from build123d import *

# Parameters (mm, degrees)
F0_W           = 101.6
F0_H           = 63.5
F1_DEPTH       = 6.35
F2_D           = 3.6576
F2_CSINK_D     = 7.7978
F2_CSINK_ANGLE = 82
F3_R           = 5.08


with BuildPart() as f1:
    # F0 (on Top) → F1 (new body)
    with BuildSketch(Plane.XY):
        Rectangle(F0_W, F0_H)
    extrude(amount=F1_DEPTH)

    # F2 (through all)
    with Locations(Plane(origin=(0, 0, 0), x_dir=(1, 0, 0), z_dir=(0, 0, -1))):
        with Locations((-13.9501372, 0), (5.0998628, 0)):
            CounterSinkHole(F2_D / 2, F2_CSINK_D / 2, counter_sink_angle=F2_CSINK_ANGLE)

    # F3
    f3_edges = [f1.edges().sort_by_distance(p)[0] for p in [
        (-50.8, -31.75, 3.175),
        (-50.8, 31.75, 3.175),
        (50.8, -31.75, 3.175),
        (50.8, 31.75, 3.175),
    ]]
    fillet(f3_edges, radius=F3_R)


solid = f1.part
The model under review builds one solid part; all positions refer to its coordinate system, in mm. Give positions to 0.01 mm unless a question says otherwise; leave off trailing zeros. Order: outer loops, then holes, each group sorted by start corner. A loop starts at its lowest first (then second) coordinate and runs counter-clockwise, first axis right, second up. Notation, with made-up numbers: (28.5, 61) -> (84.5, 61) arc R31 ccw to (84.5, 94) -> close; hole circle Ø10 at (-30, 43). An arc over 180 degrees is marked (long way). Write item = value, one per line. Start each with the question number.
(1) Take a section at A-A (y = 0). Write out the cut boundary in (x, z).
(2) Draft analysis for pull direction Y (two halves, no side actions). For faces 1 (the flat face through (-1, 0, 6.35)), 2 (the conical face through (7.027, -0.085, 2.266)), 3 (the flat face through (-1, -31.75, 3)), state which applies: +Y half, -Y half, draft (parallel to the pull), parting line (faces both ways), or undercut.
(3) For L1, parallel to Y at x = -15, z = 3.5; L2, parallel to Y at x = 47, z = 4, list the stretches that pass through material, from the lowest coordinate up. Write a range as from..to.
(4) For pin 1 Ø3.5 at (x, y) = (5.1, 0) entering from -Z; pin 2 Ø5 at (x, y) = (-13.95, 0) entering from -Z, all flat-tipped, find the tip position at first contact; note any pin that passes through.
Returned:
q1.outline = (-50.8, 0) -> (-17.85, 0) -> (-15.78, 2.38) -> (-15.78, 6.35) -> (-50.8, 6.35) -> close; (-12.12, 2.38) -> (-10.05, 0) -> (1.2, 0) -> (3.27, 2.38) -> (3.27, 6.35) -> (-12.12, 6.35) -> close; (6.93, 2.38) -> (9, 0) -> (50.8, 0) -> (50.8, 6.35) -> (6.93, 6.35) -> close
q2.face_1 = draft
q2.face_2 = undercut
q2.face_3 = -Y half
q3.L1 = -31.75..-1.5, 1.5..31.75
q3.L2 = -31.59..31.59
q4.pin_1 = through
q4.pin_2 = 1.61
